```python
from build123d import *

# Parameters (mm, degrees)
SKETCH1_W               = 30
SKETCH1_H               = 35
BOSS_EXTRUDE1_DEPTH     = 44.26
SKETCH2_W               = 26
SKETCH2_H               = 36.26
CUT_EXTRUDE1_DEPTH      = 31
CUT_EXTRUDE2_DEPTH      = 26
CUT_EXTRUDE3_DEPTH      = 64.905771257
CUT_EXTRUDE3_DEPTH_BACK = 64.905771257
SKETCH4_R               = 2.7
CUT_EXTRUDE7_DEPTH      = 62.805724654
CUT_EXTRUDE7_DEPTH_BACK = 62.805724654
SKETCH6_R               = 1.65


with BuildPart() as part:
    # Sketch1 → Boss-Extrude1 (new body)
    with BuildSketch(Plane.XY):
        with Locations((-15, 17.5)):
            Rectangle(SKETCH1_W, SKETCH1_H)
    extrude(amount=BOSS_EXTRUDE1_DEPTH)

    # Sketch2 → Cut-Extrude1 (cut)
    with BuildSketch(Plane(origin=(0, 35, 0), x_dir=(1, 0, 0), z_dir=(0, 1, 0))):
        with Locations((-17, -22.13)):
            Rectangle(SKETCH2_W, SKETCH2_H)
    extrude(amount=-CUT_EXTRUDE1_DEPTH, mode=Mode.SUBTRACT)

    # Sketch3 → Cut-Extrude2 (cut)
    with BuildSketch(Plane.ZY.offset(30)):
        with BuildLine():
            Line((4, 27.602220032), (4, 22.397779968))
            ThreePointArc((4, 22.397779968), (1.570379812, 22.680763567), (2.347731949, 25))
            ThreePointArc((2.347731949, 25), (1.570379812, 27.319236433), (4, 27.602220032))
        make_face()
        with BuildLine():
            Line((40.26, 27.602220032), (40.26, 22.397779968))
            ThreePointArc((40.26, 22.397779968), (42.689620188, 22.680763567), (41.912268051, 25))
            ThreePointArc((41.912268051, 25), (42.689620188, 27.319236433), (40.26, 27.602220032))
        make_face()
    extrude(amount=-CUT_EXTRUDE2_DEPTH, mode=Mode.SUBTRACT)

    # Sketch4 → Cut-Extrude3 (cut, two sides: drawn at the far end of the back side and taken through both)
    with BuildSketch(Plane(origin=(0, 0, 0), x_dir=(0, 0, -1), z_dir=(1, 0, 0)).offset(-CUT_EXTRUDE3_DEPTH_BACK)):
        with Locations(Location((-22.13, 25, 0), (0, 0, 90))):
            Circle(SKETCH4_R)
    extrude(amount=CUT_EXTRUDE3_DEPTH + CUT_EXTRUDE3_DEPTH_BACK, mode=Mode.SUBTRACT)

    # Sketch6 → Cut-Extrude7 (cut, two sides: drawn at the far end of the back side and taken through both)
    with BuildSketch(Plane(origin=(0, 4, 0), x_dir=(1, 0, 0), z_dir=(0, 1, 0)).offset(-CUT_EXTRUDE7_DEPTH_BACK)):
        with Locations(Location((-24, -34.26, 0), (0, 0, 180))):
            Circle(SKETCH6_R)
        with Locations(Location((-12, -34.26, 0), (0, 0, 180))):
            Circle(SKETCH6_R)
        with Locations((-12, -14.26)):
            Circle(SKETCH6_R)
        with Locations((-24, -14.26)):
            Circle(SKETCH6_R)
    extrude(amount=CUT_EXTRUDE7_DEPTH + CUT_EXTRUDE7_DEPTH_BACK, mode=Mode.SUBTRACT)


solid = part.part
```
Could you check a few things on this model? Use its own coordinates, in mm. A direction names the side the tool comes from. Coordinates: 2 decimals unless noted, no trailing zeros. Write each loop counter-clockwise with the first axis right and the second up, starting at its lowest first coordinate (ties: lowest second). Pieces come first, ordered by that corner, then holes. Notation, with made-up numbers: (33.5, -34) -> (51.5, -34) arc R19 cw to (51.5, -14) -> close; hole circle Ø8 at (-34, -1.75). An arc over 180 degrees is marked (long way). Return JSON: item names as keys, results as strings.
(1) Which directions (+Z, -Z, +X, -X, +Y, -Y) give clear straight access to the entire face, cutting with the end or side of a thin tool? Please do faces 4 (the flat face through (-17, 13, 4)), 5 (the flat face through (-30, 3, 20)), 6 (the cylindrical face through (-17.18, 22.65, 42.67)).
Numbers:
{"face 4": "-X, +Y", "face 5": "+Z, -Z, -X, +Y, -Y", "face 6": "-X"}
(2) Imagine slicing it at D-D, the plane y = 30. Please give me the cut outline in (x, z), then the cut area to 3 significant figures.
Numbers:
{"outline": "(-30, 0) -> (0, 0) -> (0, 44.26) -> (-30, 44.26) -> (-30, 40.26) -> (-4, 40.26) -> (-4, 4) -> (-30, 4) -> close", "area": "385 mm2"}
(3) Imagine slicing it at A-A, the plane z = 14.26. Please give me the cut outline in (x, y), then the cut area to 3 significant figures.
Numbers:
{"outline": "(-30, 0) -> (-25.65, 0) -> (-25.65, 4) -> (-30, 4) -> close; (-22.35, 0) -> (-13.65, 0) -> (-13.65, 4) -> (-22.35, 4) -> close; (-10.35, 0) -> (0, 0) -> (0, 35) -> (-4, 35) -> (-4, 4) -> (-10.35, 4) -> close", "area": "218 mm2"}
(4) Imagine slicing it at B-B, the plane z = 22.13. Please give me the cut outline in (x, y).
Numbers:
{"outline": "(-30, 0) -> (0, 0) -> (0, 22.3) -> (-4, 22.3) -> (-4, 4) -> (-30, 4) -> close; (-4, 27.7) -> (0, 27.7) -> (0, 35) -> (-4, 35) -> close"}
(5) We'd pull the mould along Y, two halves only. Please class faces 1 (the cylindrical face through (-2, 24.6, 24.8)), 2 (the flat face through (-17, 4, 22)), 3 (the cylindrical face through (-11.11, 1.97, 12.87)): +Y half, -Y half, draft (parallel to the pull), parting line (faces both ways), or undercut.
Numbers:
{"face 1": "undercut", "face 2": "+Y half", "face 3": "draft"}
(6) I need wall thicknesses on L1, parallel to Z at x = -12, y = 1.45; L2, parallel to Z at x = -12, y = 12; L3, parallel to Z at x = -3, y = 25. Which ranges of each line are inside material? Lowest first, please.
Numbers:
{"L1": "z = 0 to 12.61, 15.91 to 32.61, 35.91 to 44.26", "L2": "z = 0 to 4, 40.26 to 44.26", "L3": "z = 0 to 19.43, 24.83 to 44.26"}
(7) I'm going to push flat-ended pins straight in: pin 1 (6 mm diameter, centred on y = 25.5, z = 29.5, fed in from -X); pin 2 (1 mm diameter, centred on x = -16.5, z = 33, fed in from +Y). Where does each tip first touch, or does it pass through?
Numbers:
{"pin 1": "stops at x = -4", "pin 2": "stops at y = 4"}
(8) Imagine slicing it at C-C, the plane x = -13. Please give me the cut outline in (y, z) (3 decimals).
Numbers:
{"outline": "(0, 0) -> (35, 0) -> (35, 4) -> (27.602, 4) arc R1.575 cw (long way) to (25, 2.348) arc R1.575 cw (long way) to (22.398, 4) -> (4, 4) -> (4, 12.948) -> (0, 12.948) -> close; (0, 15.572) -> (4, 15.572) -> (4, 32.948) -> (0, 32.948) -> close; (0, 35.572) -> (4, 35.572) -> (4, 40.26) -> (22.398, 40.26) arc R1.575 cw (long way) to (25, 41.912) arc R1.575 cw (long way) to (27.602, 40.26) -> (35, 40.26) -> (35, 44.26) -> (0, 44.26) -> close"}
